Part model, mm, in its own coordinate system. A direction names the side the tool comes from. Give positions to 0.01 mm unless a question says otherwise; leave off trailing zeros. Order: outer loops, then holes, each group sorted by start corner. A loop starts at its lowest first (then second) coordinate and runs counter-clockwise, first axis right, second up.
1. Drop flat-ended pins along their axis: pin 1 Ø3 at (x, y) = (5, 2) entering from -Z; pin 2 Ø6 at (x, y) = (3.5, 4.5) entering from -Z; pin 3 Ø5 at (y, z) = (6.5, 33.5) entering from +X. Give the stop position or say it passes through.
2. Slice it at B-B on x = 5.5. List the corners of the cut face in (y, z), and give its area (3 significant figures).
3. Slice it at C-C on y = 7.5. List the corners of the cut face in (x, z), and give its area (3 significant figures).
4. Which spindle directions (+Z, -Z, +X, -X, +Y, -Y) get a long thin tool onto all of the face, cutting with end or side? Do faces 1 (the flat face through (6, 2, 104)), 2 (the flat face through (1.6, 7.7, 208.4)). Say none if no direction does.
5. Slice it at A-A on z = 180. List the corners of the cut face in (x, y).
6. Probe line 1 (X direction, y = 15, z = 19); line 2 (Z direction, x = 1, y = 14.5). List the from-to ranges inside material, lowest first.
Autodesk Inventor part; units mm, degrees
ref_plane "YZ Plane" through (0, 0, 0) normal (1, 0, 0) x (0, 1, 0)
ref_plane "XZ Plane" through (0, 0, 0) normal (0, 1, 0) x (-1, 0, 0)
ref_plane "XY Plane" through (0, 0, 0) normal (0, 0, 1) x (1, 0, 0)
sketch "Szkic1" plane through (0, 0, 0) normal (0, 0, 1) x (1, 0, 0)
  line L0 (-2.2485, 0) -> (12.0414, 0)
  line L1 (0, -4.2485) -> (0, 24.0414)
  line L2 (10, 0) -> (1, 0)
  line L3 (0, 1) -> (0, 20)
  line L4 (2, 20) -> (2, 3)
  line L5 (3, 2) -> (10, 2)
  line L6 (0, 20) -> (2, 20)
  line L7 (10, 0) -> (10, 2)
  arc A0 (2, 3) -> (3, 2) centre (3, 3) ccw
  arc A1 (0, 1) -> (1, 0) centre (1, 1) ccw
  point P0 (0, 0)
  dimension "d0" = 20
  dimension "d1" = 10
  dimension "d2" = 2
  dimension "d3" = 1
extrude "Wyciągnięcie proste1" add sketch "Szkic1" along normal blind 210 contours A1 L1 L6 L4 A0 L5 L7 L0
sketch "Szkic2" plane through (1, 0, 0) normal (0, -1, 0) x (1, 0, 0)
  line L0 (0, 0) -> (9, 0)
  line L1 (9, 0) -> (9, 210)
  line L2 (0, 210) -> (9, 210)
  line L3 (-1, 0) -> (-1, 210)
  line L4 (-1, 210) -> (9, 200)
  line L5 (9, 200) -> (9, 210)
  line L6 (9, 210) -> (-1, 210)
  line L7 (-1, 0) -> (9, 10)
  line L8 (9, 10) -> (9, 0)
  line L9 (9, 0) -> (-1, 0)
  dimension "d6" = 135
  dimension "d7" = 45
extrude "Wyciągnięcie proste2" cut sketch "Szkic2" against normal through all contours L9 L7 L1 L0 | L6 L2 L1 L4
properties part number "kątownik_mały2" material "Aluminium 6061"
Data:
1. pin 1: stops at z = 3.5
1. pin 2: stops at z = 0.5
1. pin 3: stops at x = 2
2. outline: (0, 5.5) - (2, 5.5) - (2, 204.5) - (0, 204.5) - close
2. area: 398 mm2
3. outline: (0, 0) - (2, 2) - (2, 208) - (0, 210) - close
3. area: 416 mm2
4. face 1: +Z, -Z, +X, +Y
4. face 2: +Z, +X, +Y, -Y
5. outline: (0, 1) arc R1 ccw to (1, 0) - (10, 0) - (10, 2) - (3, 2) arc R1 cw to (2, 3) - (2, 20) - (0, 20) - close
6. line 1: x = 0 to 2
6. line 2: z = 1 to 209
